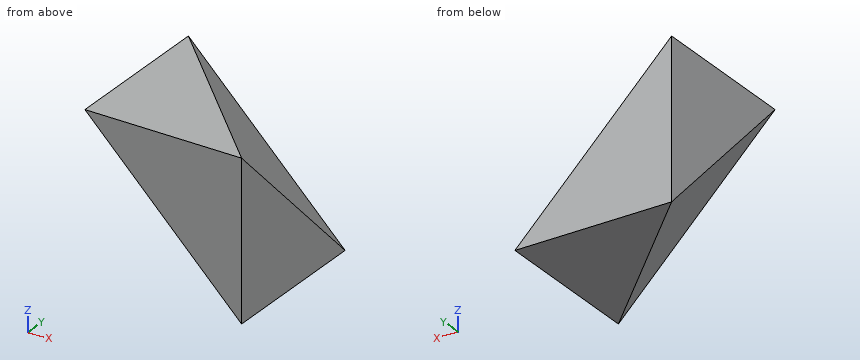
from build123d import *

# Parameters (mm, degrees)
SKETCH1_W           = 80
SKETCH1_H           = 80
BOSS_EXTRUDE1_DEPTH = 80
CUT_EXTRUDE1_DEPTH  = 80
CUT_EXTRUDE2_DEPTH  = 80


with BuildPart() as part:
    # Sketch1 → Boss-Extrude1 (new body)
    with BuildSketch(Plane(origin=(0, 0, 0), x_dir=(1, 0, 0), z_dir=(0, 1, 0))):
        Rectangle(SKETCH1_W, SKETCH1_H)
    extrude(amount=BOSS_EXTRUDE1_DEPTH)

    # Sketch5 → Cut-Extrude1 (cut)
    with BuildSketch(Plane(origin=(26.666666667, 26.666666667, 26.666666667), x_dir=(0.8164965809277261, -0.40824829046386296, -0.4082482904638629), z_dir=(0.5773502691896256, 0.5773502691896263, 0.5773502691896254))):
        Polygon((-81.649658093, 28.284271247), (16.329931619, -28.284271247), (16.329931619, 84.852813742), align=None)
    extrude(amount=CUT_EXTRUDE1_DEPTH, mode=Mode.SUBTRACT)

    # Sketch6 → Cut-Extrude2 (cut)
    with BuildSketch(Plane(origin=(0, 0, 0), x_dir=(0.8164965809277261, -0.40824829046386296, -0.4082482904638629), z_dir=(0.5773502691896256, 0.5773502691896263, 0.5773502691896254))):
        Polygon((-48.989794856, -28.284271247), (48.989794856, 28.284271247), (-48.989794856, 84.852813742), align=None)
    extrude(amount=-CUT_EXTRUDE2_DEPTH, mode=Mode.SUBTRACT)


solid = part.part
Geometry check sheet. Reference: the model listing, model coordinates, mm. Coordinates: 2 decimals unless noted, no trailing zeros. Write each loop counter-clockwise with the first axis right and the second up, starting at its lowest first coordinate (ties: lowest second). Pieces come first, ordered by that corner, then holes. Notation, with made-up numbers: (31, -27) -> (86, -27) arc R25 cw to (86, 11) -> close; hole circle Ø9 at (83.5, 38). An arc over 180 degrees is marked (long way). One line per question, with ' | ' between items.
1. Cross-section at A-A on y = 19. Record the cut outline in (x, z), and give its area (3 significant figures).
Answers:
outline: (-40, 21) -> (21, -40) -> (40, -40) -> (40, 21) -> (21, 40) -> (-40, 40) -> close | area: 4,360 mm²
2. Cross-section at B-B on x = -5. Record the cut outline in (y, z), and give its area (4 significant figures).
Answers:
outline: (0, 5) -> (45, -40) -> (80, -40) -> (80, 5) -> (45, 40) -> (0, 40) -> close | area: 4,775 mm²
3. Depth check by flat-ended pin: pin 1 Ø1 at (x, z) = (-12.5, 6) entering from -Y; pin 2 Ø3 at (x, z) = (26, 27) entering from +Y; pin 3 Ø5 at (x, z) = (-3, -21.5) entering from -Y. Enter the tip coordinate at first touch or a pass-through.
Answers:
pin 1: stops at y = 5.79 | pin 2: stops at y = 29.12 | pin 3: stops at y = 20.96
4. Thickness scan on probe 1 along Z at (x, y) = (11.5, 63); probe 2 along X at (y, z) = (26.5, 27.5); probe 3 along Z at (x, y) = (3, 16). Record the ranges inside material, lowest first. Write a range as from..to.
Answers:
probe 1: z = -40..5.5 | probe 2: x = -40..26 | probe 3: z = -19..40
